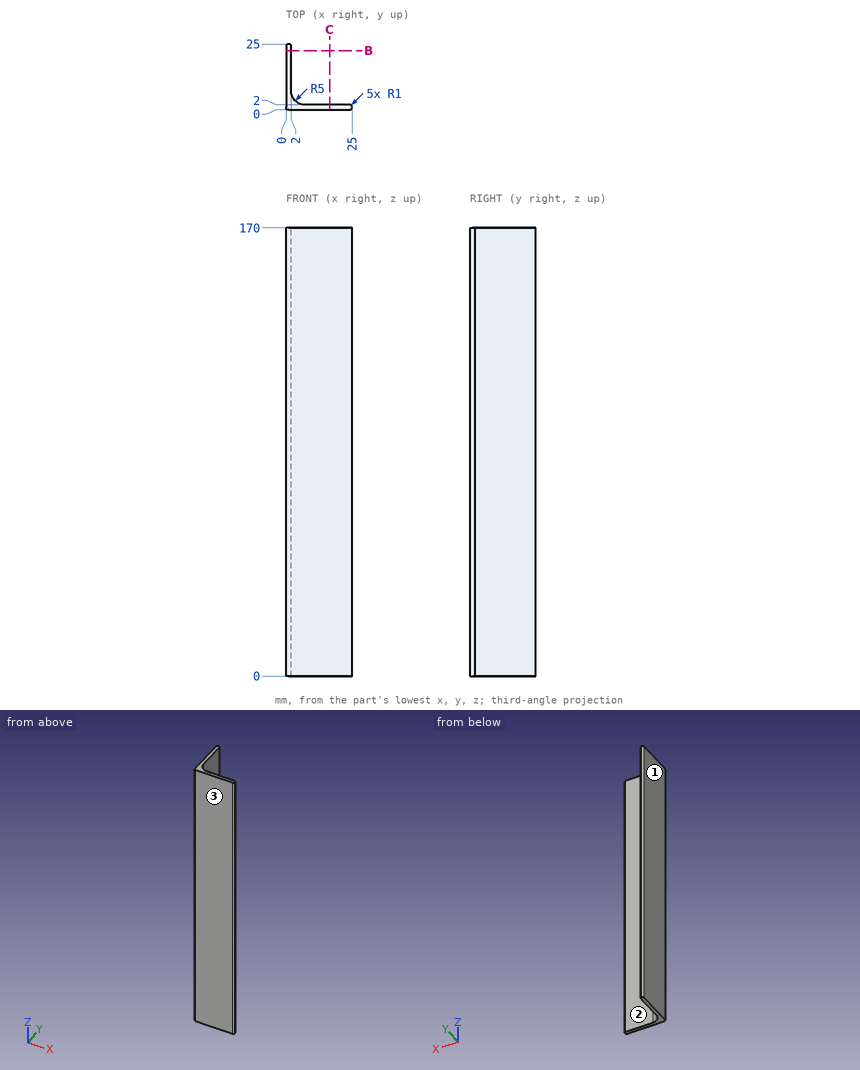
Answer from the drawing. Dimensions are ordinates in mm from the lowest x, y and z of the part. Give positions to 0.01 mm unless a question says otherwise; leave off trailing zeros. Loops run counter-clockwise (first coordinate to the right, second up) from the corner with the lowest first, then second, coordinate; pieces in that order, holes last. Notation, with made-up numbers: (37, 30.25) - (59, 30.25) arc R20 cw to (59, 60.25) - close; hole circle Ø2 at (88.25, 17). An arc over 180 degrees is marked (long way). Answer as CSV lines item,"result". Start each with the question number.
Item 1: Find the intervals of material crossed by line 1 (X direction, y = 22.5, z = 61.5); line 2 (Y direction, x = 4, z = 119), in increasing order. Write a range as from..to.
Item 2: The mould has two halves that part along Y. Classify the marked faces 1, 2 and 3: +Y half, -Y half, draft (parallel to the pull), parting line (faces both ways), or undercut.
Item 3: Each of these flat-tipped pins is pushed along its axis until it touches: pin 1 (8.5 mm diameter, centred on x = 13, z = 107.5, fed in from +Y); pin 2 (5 mm diameter, centred on y = 14, z = 120.5, fed in from +X); pin 3 (5 mm diameter, centred on y = 14.5, z = 118.5, fed in from -X); pin 4 (5 mm diameter, centred on y = 8, z = 141.5, fed in from +X). Where does it stop, or does it pass through?
Item 4: A cutting plane is placed at B-B on y = 22.5. Determine the outline of the cut face in (x, z), then the cut area to 3 significant figures.
Found:
1,line 1,"x = 0..2"
1,line 2,"y = 0..3"
2,face 1,"draft"
2,face 2,"+Y half"
2,face 3,"-Y half"
3,pin 1,"stops at y = 2"
3,pin 2,"stops at x = 2"
3,pin 3,"stops at x = 0"
3,pin 4,"stops at x = 2.23"
4,outline,"(0, 0) - (2, 0) - (2, 170) - (0, 170) - close"
4,area,"340 mm^2"
